Source: three-view drawing plus pictorial views. Frame: mm from the lowest corner of the part. A direction names the side the tool comes from. Coordinates: 2 decimals unless noted, no trailing zeros. Loops run counter-clockwise (first coordinate to the right, second up) from the corner with the lowest first, then second, coordinate; pieces in that order, holes last.
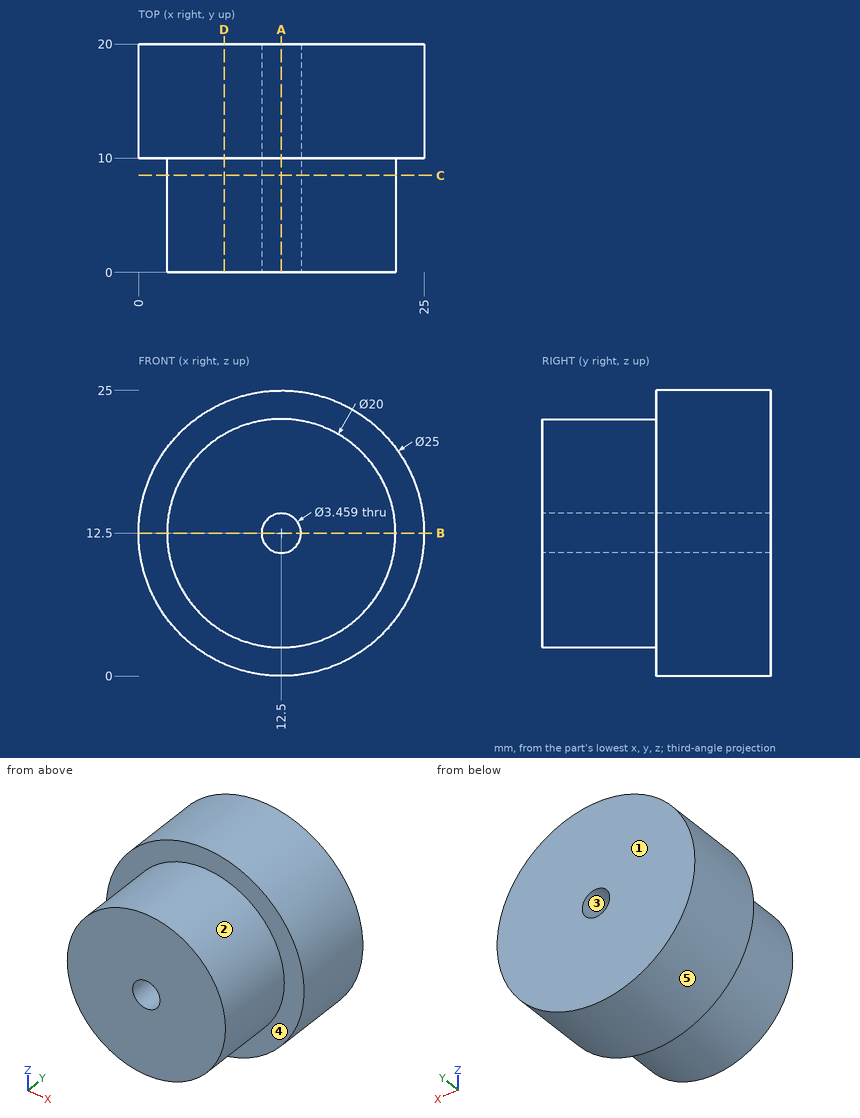
Q1. Material intervals for line 1 along Z through (x, y) = (12.5, 6); line 2 along Z through (x, y) = (12.5, 12.25); line 3 along Y through (x, z) = (8, 23.75), sorted ascending.
Q2. First-contact query: pin 1 Ø12.5 at (x, z) = (6.5, 11) entering from -Y; pin 2 Ø5 at (x, y) = (21.5, 8.5) entering from -Z; pin 3 Ø2 at (x, z) = (12.5, 12.5) entering from +Y; pin 4 Ø5 at (x, y) = (22, 10.5) entering from -Z. Flat tips, straight axial feed; report the tip coordinate or a pass-through.
Q3. Reachability of the marked faces 1 and 2 from +Z, -Z, +X, -X, +Y, -Y: full face, straight path, thin tool, end or side. Return the list, or none.
Q4. Section query C-C on y = 8.5. Return the cut outline in (x, z).
Q5. Section query D-D on x = 7.5. Return the cut outline in (y, z), then the cut area to 3 significant figures.
Q6. Section query B-B on z = 12.5. Return the cut outline in (x, y).
Q7. Section query A-A on x = 12.5. Return the cut outline in (y, z).
Q8. Draft query along Z for the marked faces 3, 4 and 5. Return one class per face: released by +Z, released by -Z, zero draft, split by the parting line, or undercut.
Resolved:
1. line 1: z = 2.5 to 10.77, 14.23 to 22.5
1. line 2: z = 0 to 10.77, 14.23 to 25
1. line 3: y = 10 to 20
2. pin 1: stops at y = 0
2. pin 2: stops at z = 2.14
2. pin 3: passes through
2. pin 4: stops at z = 2.14
3. face 1: +Z, -Z, +X, -X, +Y
3. face 2: -Y
4. outline: circle Ø20 at (12.5, 12.5); hole circle Ø3.46 at (12.5, 12.5)
5. outline: (0, 3.84) - (10, 3.84) - (10, 1.04) - (20, 1.04) - (20, 23.96) - (10, 23.96) - (10, 21.16) - (0, 21.16) - close
5. area: 402 mm2
6. outline: (0, 10) - (2.5, 10) - (2.5, 0) - (10.77, 0) - (10.77, 20) - (0, 20) - close; (14.23, 0) - (22.5, 0) - (22.5, 10) - (25, 10) - (25, 20) - (14.23, 20) - close
7. outline: (0, 2.5) - (10, 2.5) - (10, 0) - (20, 0) - (20, 10.77) - (0, 10.77) - close; (0, 14.23) - (20, 14.23) - (20, 25) - (10, 25) - (10, 22.5) - (0, 22.5) - close
8. face 3: undercut
8. face 4: zero draft
8. face 5: split by the parting line
